Geometry check sheet. Reference: the model listing, model coordinates, mm. A direction names the side the tool comes from. Coordinates: 2 decimals unless noted, no trailing zeros. Write each loop counter-clockwise with the first axis right and the second up, starting at its lowest first coordinate (ties: lowest second). Pieces come first, ordered by that corner, then holes. Notation, with made-up numbers: (46, -22) -> (72, -22) arc R16 ccw to (72, -9) -> close; hole circle Ø1 at (35.25, -3.5). An arc over 180 degrees is marked (long way). Answer in a Markdown table with one row per item. Add a question column.
Q1. Tool access check on faces 4 (the face through (45, 0, 28)), 5 (the face through (-38.06, -0.91, 18.87)), 6 (the face through (-13, 13, 0)). Record the directions out of +Z, -Z, +X, -X, +Y, -Y that give a thin tool (end or side, any length) a straight path to the whole face; none if there is none.
Q2. Gauge pin test, flat ends, axial feed: P1, Ø4, axis at x = 7.5, y = 17, coming from the +Z side; P2, Ø10, axis at x = 10, z = 20, coming from the +Y side; P3, Ø4, axis at x = 20, z = 10.5, coming from the +Y side; P4, Ø1.5, axis at x = 22, z = -2, coming from the +Y side. Record the tip position at first contact, or that the pin passes through.
Q3. Release check for a two-part mould opening along X. For faces 1 (the face through (25.61, -35.05, 18.87)), 2 (the face through (13.887, 10.648, -19.72)), 3 (the face through (32, -32, 28)) record: pulls with the +X half, pulls with the -X half, needs draft (parallel to the pull), parting line crosses it, or undercut.
Q4. Thickness scan on line 1 (Y direction, x = -0.5, z = 17); line 2 (Z direction, x = -13, y = -32); line 3 (Z direction, x = -4.5, y = -46). Record the ranges inside material, lowest first.
Q5. Section check C-C, the plane x = 11. Record the boundary of the cut face in (y, z), and give its area (3 significant figures).
Q6. Section check A-A, the plane y = 0. Record the boundary of the cut face in (x, z), and give its area (3 significant figures).
Q7. Section check D-D, the plane z = 5. Record the boundary of the cut face in (x, y).
Autodesk Inventor part; units mm, degrees
ref_plane "YZ Plane" through (0, 0, 0) normal (1, 0, 0) x (0, 1, 0)
ref_plane "XZ Plane" through (0, 0, 0) normal (0, 1, 0) x (-1, 0, 0)
ref_plane "XY Plane" through (0, 0, 0) normal (0, 0, 1) x (1, 0, 0)
sketch "스케치1" plane through (0, 0, 0) normal (0, 0, 1) x (1, 0, 0)
  circle A0 centre (0, 0) radius 55
  dimension "d0" = 110
extrude "돌출1" add sketch "스케치1" along normal blind 10
sketch "스케치2" plane through (0, 0, 10) normal (0, 0, 1) x (1, 0, 0)
  circle A0 centre (0, 0) radius 45 construction
  line L0 (0, 0) -> (0, 45) construction
  circle A1 centre (0, 45) radius 7
  dimension "d3" = 90
  dimension "d4" = 14
extrude "돌출2" add sketch "스케치2" along normal blind 18
pattern_circular "원형 패턴1" count 8 over 360 about axis through (0, 0, 0) along (0, 0, 1) of "돌출2"
sketch "스케치3" plane through (0, 0, 0) normal (0, 0, -1) x (-1, 0, 0)
  circle A0 centre (0, 0) radius 17.5
  dimension "d10" = 35
extrude "돌출3" add sketch "스케치3" along normal blind 40
properties part number "out_shaft"
Calculated:
| question | item | result |
|---|---|---|
| 1 | face 4 | +Z, +X, -X, +Y, -Y |
| 1 | face 5 | +Z |
| 1 | face 6 | -Z |
| 2 | P1 | stops at z = 10 |
| 2 | P2 | stops at y = 49.9 |
| 2 | P3 | stops at y = 51.95 |
| 2 | P4 | passes through |
| 3 | face 1 | undercut |
| 3 | face 2 | parting line crosses it |
| 3 | face 3 | needs draft |
| 4 | line 1 | y = -51.98 to -38.02, 38.02 to 51.98 |
| 4 | line 2 | z = 0 to 10 |
| 4 | line 3 | z = 0 to 28 |
| 5 | outline | (-53.89, 0) -> (-13.61, 0) -> (-13.61, -40) -> (13.61, -40) -> (13.61, 0) -> (53.89, 0) -> (53.89, 10) -> (-53.89, 10) -> close |
| 5 | area | 2,170 mm² |
| 6 | outline | (-55, 0) -> (-17.5, 0) -> (-17.5, -40) -> (17.5, -40) -> (17.5, 0) -> (55, 0) -> (55, 10) -> (52, 10) -> (52, 28) -> (38, 28) -> (38, 10) -> (-38, 10) -> (-38, 28) -> (-52, 28) -> (-52, 10) -> (-55, 10) -> close |
| 6 | area | 3,000 mm² |
| 7 | outline | circle Ø110 at (0, 0) |
